Solid Edge part; units mm, degrees
sketch "Sketch1" plane through (0, 0, 0) normal (1, 0, 0) x (0, 1, 0)
  line L0 (0, 0) -> (0, -12)
  line L1 (0, -12) -> (-12, -12)
  line L2 (-12, -12) -> (-12, -4)
  line L3 (-12, -4) -> (-20, -4)
  line L4 (-20, -4) -> (-20, 6)
  line L5 (-20, 6) -> (6, 6)
  line L6 (6, 6) -> (6, 0)
  line L7 (6, 0) -> (0, 0)
  dimension "D1" = 6
  dimension "D2" = 6
  dimension "D3" = 12
  dimension "D4" = 12
extrude "Protrusion1" add sketch "Sketch1" along normal mid plane 20
chamfer "Chamfer_1" distance 8 angle 45 1 edges at (0, -12, -4)
hole "Hole_1" at (0, -20, -8) direction (0, 1, 0) diameter 5.8 end up to next counterbore diameter 10 counterbore depth 5.8
hole "Hole_2" at (-5, -15, 6) direction (0, 0, -1) diameter 3.75 depth 10 tip angle 118 start chamfer 0.6 start chamfer angle 30 end chamfer 0.6 end chamfer angle 30
pattern_linear "Pattern1" count 2 spacing 10 along (1, 0, 0) count 2 spacing 10 along (0, 1, 0) of "Hole_2"
sketch "Sketch2" plane through (0, -7, 6) normal (0, 0, 1) x (-1, 0, 0)
  line L0 (-10, 1.5) -> (10, 1.5)
  line L1 (10, 1.5) -> (10, 4.5)
  line L2 (10, 4.5) -> (-10, 4.5)
  line L3 (-10, 4.5) -> (-10, 1.5)
extrude "ExtrudedCutout_1" cut sketch "Sketch2" against normal blind 5
properties material "Polyethylene, low density"
Model file for the job. Use its own axes, mm. A direction names the side the tool comes from. Round coordinates to 2 decimals unless told otherwise and drop trailing zeros. Order: outer loops, then holes, each group sorted by start corner. A loop starts at its lowest first (then second) coordinate and runs counter-clockwise, first axis right, second up. Notation, with made-up numbers: M 67.25,-22.5 L 90.25,-22.5 A21 cw 90.25,9.5 Z; hole C 66,2.5 d4. An arc over 180 degrees is marked long. Write each question's results on one line, items separated by ' | '. Start each with the question number.
(1) Saw through at C-C, the plane z = -9. Give the cut face in (x, y), then the cut area to 3 significant figures.
(2) Saw through at A-A, the plane z = -2.25. Give the cut face in (x, y) (3 decimals), then the cut area to 3 significant figures.
(3) Drop flat-ended pins along their axis: pin 1 (5 mm diameter, centred on x = -4, y = 4.5, fed in from -Z); pin 2 (6 mm diameter, centred on x = 0.5, z = -5.5, fed in from +Y); pin 3 (8 mm diameter, centred on x = -7.5, y = 2.5, fed in from -Z); pin 4 (2 mm diameter, centred on x = -1, z = -6, fed in from -Y). Give the stop position or say it passes through.
(4) Saw through at D-D, the plane y = 3. Give the cut face in (x, z), then the cut area to 3 significant figures.
(5) Probe probe 1 along Y at (x, z) = (5, -0.75) (3 decimals); probe 2 along X at (y, z) = (-5, 0.75) (3 decimals); probe 3 along Y at (x, z) = (5, 1.5) (3 decimals). List the from-to ranges inside material, lowest first. Write a range as from..to.
(6) Two-plate mould, pull along X, no slides. Class faces 1 (the face through (3.73, -13.62, 0.42)), 2 (the face through (0, -10, 1)), 3 (the face through (10, -7, -3)): pulls with the +X half, pulls with the -X half, needs draft (parallel to the pull), parting line crosses it, or undercut.
(7) Which spindle directions (+Z, -Z, +X, -X, +Y, -Y) get a long thin tool onto all of the face, cutting with end or side? Do faces 4 (the face through (0, 3, 0)), 5 (the face through (0, -6, -12)), 6 (the face through (0, -8.5, 4)). Say none if no direction does.
Established:
1) outline: M -10,-15 L -4.9,-15 L -4.9,-14.2 L -2.72,-14.2 L -2.72,0 L -10,0 Z; M 2.72,-14.2 L 4.9,-14.2 L 4.9,-15 L 10,-15 L 10,0 L 2.72,0 Z | area: 215 mm^2
2) outline: M -10,-20 L 10,-20 L 10,0 L -10,0 Z; hole C -5,-15 d3.75; hole C -5,-5 d3.75; hole C 5,-15 d3.75; hole C 5,-5 d3.75 | area: 356 mm^2
3) pin 1: stops at z = 0 | pin 2: stops at y = 0 | pin 3: stops at z = -12 | pin 4: stops at y = -14.2
4) outline: M -10,0 L 10,0 L 10,6 L -10,6 Z | area: 120 mm^2
5) probe 1: y = -20..-16.875, -13.125..-6.875, -3.125..0 | probe 2: x = -10..-6.875, -3.125..3.125, 6.875..10 | probe 3: y = -20..-16.875, -13.125..-11.5, -8.5..-6.875, -3.125..6
6) face 1: undercut | face 2: needs draft | face 3: pulls with the +X half
7) face 4: -Z, +X, -X, +Y | face 5: -Z, +X, -X, +Y, -Y | face 6: +Z, +X, -X
